Part print with two shaded views. Sizes in mm from the minimum x, y, z corner. A direction names the side the tool comes from. Give positions to 0.01 mm unless a question says otherwise; leave off trailing zeros. Order: outer loops, then holes, each group sorted by start corner. A loop starts at its lowest first (then second) coordinate and runs counter-clockwise, first axis right, second up.
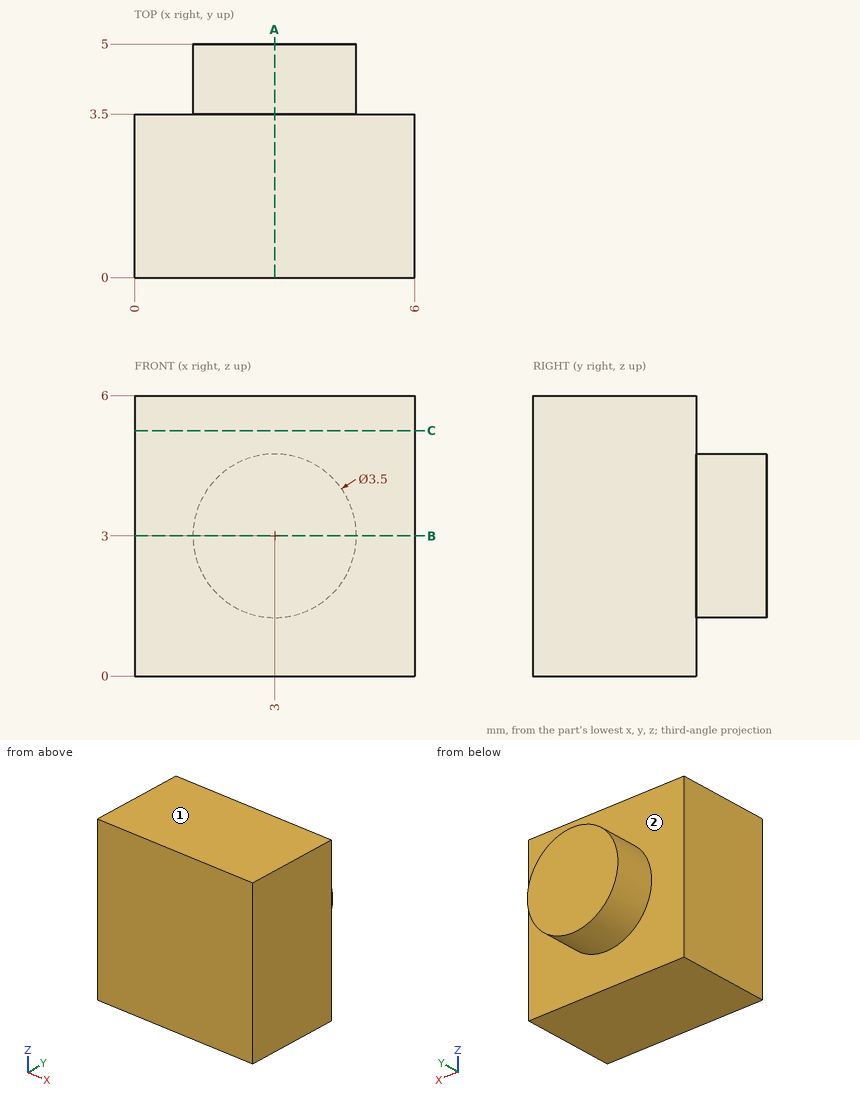
Item 1: Slice it at C-C (z = 5.25). Give the cut face in (x, y).
Item 2: Tool access for the marked faces 1 and 2: list every direction of +Z, -Z, +X, -X, +Y, -Y with a clear straight run to the whole face (end or side of a thin tool).
Item 3: Slice it at A-A (x = 3). Give the cut face in (y, z), and give its area (4 significant figures).
Item 4: Wall check: L1, parallel to Y at x = 0.85, z = 5; L2, parallel to Z at x = 1.4, y = 4; L3, parallel to Z at x = 3.2, y = 4.6. Give the ranges that are in metal, low to high.
Item 5: Slice it at B-B (z = 3). Give the cut face in (x, y), and give its area (4 significant figures).
A:
1. outline: (0, 0) - (6, 0) - (6, 3.5) - (0, 3.5) - close
2. face 1: +Z, +X, -X, +Y, -Y
2. face 2: +Y
3. outline: (0, 0) - (3.5, 0) - (3.5, 1.25) - (5, 1.25) - (5, 4.75) - (3.5, 4.75) - (3.5, 6) - (0, 6) - close
3. area: 26.25 mm2
4. L1: y = 0 to 3.5
4. L2: z = 2.29 to 3.71
4. L3: z = 1.26 to 4.74
5. outline: (0, 0) - (6, 0) - (6, 3.5) - (4.75, 3.5) - (4.75, 5) - (1.25, 5) - (1.25, 3.5) - (0, 3.5) - close
5. area: 26.25 mm2
